CAD build for the part. Positions are in the model's coordinates, mm. A direction names the side the tool comes from. Give positions to 0.01 mm unless a question says otherwise; leave off trailing zeros. Loops run counter-clockwise (first coordinate to the right, second up) from the corner with the lowest first, then second, coordinate; pieces in that order, holes last. Notation, with made-up numbers: M 49.25,34 L 104.25,34 A22 ccw 104.25,52 Z; hole C 71.5,37 d2. An arc over 180 degrees is marked long. One line per question, with ' | ' between items.
```python
from build123d import *

# Parameters (mm, degrees)
F0_W      = 69.85
F0_H      = 76.2
F1_DEPTH  = 20.32
F2_R      = 5.08
F3_R      = 2.3749
F4_DEPTH  = 20.321
F5_R      = 10.0274789958
F6_DEPTH  = 8.128
F7_R      = 6.9469
F8_DEPTH  = 0.508
F10_DEPTH = 17.145
F11_R     = 10.9855
F12_DEPTH = 5.08
F11_R_2   = 5.08
F13_DEPTH = 6.35
F14_DEPTH = 6.35
F15_R     = 1.905
F16_DEPTH = 5.08
F18_R     = 1.927412261
F18_R_2   = 1.8880097215
F19_DEPTH = 3.048
F21_DEPTH = 76.2
F22_R     = 10.16
F23_DEPTH = 13.208
F25_DEPTH = 7.62
F27_DEPTH = 6.35


with BuildPart() as f1:
    # F0 (on Front) → F1 (new body)
    with BuildSketch(Plane.XZ):
        Rectangle(F0_W, F0_H)
    extrude(amount=F1_DEPTH)

    # F2
    f2_edges = [f1.edges().sort_by_distance(p)[0] for p in [
        (-34.925, -10.16, 38.1),
        (-34.925, -10.16, -38.1),
        (34.925, -10.16, -38.1),
        (34.925, -10.16, 38.1),
    ]]
    fillet(f2_edges, radius=F2_R)

    # F3 (on face) → F4 (cut, through all)
    with BuildSketch(Plane.XZ.offset(20.32)):
        with Locations((-29.845, 33.02)):
            Circle(F3_R)
        with Locations((29.845, 33.02)):
            Circle(F3_R)
        with Locations((-29.845, -33.02)):
            Circle(F3_R)
        with Locations((29.845, -33.02)):
            Circle(F3_R)
    extrude(amount=-F4_DEPTH, mode=Mode.SUBTRACT)

    # F5 (on face) → F6 (join)
    with BuildSketch(Plane.XZ.offset(20.32)):
        with Locations((0, 15.24)):
            Circle(F5_R)
    extrude(amount=F6_DEPTH)

    # F7 (on face) → F8 (cut)
    with BuildSketch(Plane.XZ.offset(28.448)):
        with Locations((0, 15.24)):
            Circle(F7_R)
    extrude(amount=-F8_DEPTH, mode=Mode.SUBTRACT)

    # F9 (on face) → F10 (join)
    with BuildSketch(Plane.XZ.offset(27.94)):
        with BuildLine():
            Line((2.3486417351, 18.4785), (-2.3486417351, 18.4785))
            ThreePointArc((-2.3486417351, 18.4785), (0, 11.2395), (2.3486417351, 18.4785))
        make_face()
    extrude(amount=F10_DEPTH)

    # F11 (on face) → F12 (join)
    with BuildSketch(Plane(origin=(0, 0, 0), x_dir=(-1, 0, 0), z_dir=(0, 1, 0))):
        with Locations((0, -22.86)):
            Circle(F11_R)
    extrude(amount=F12_DEPTH)

    # F11 (on face) → F13 (join)
    with BuildSketch(Plane(origin=(0, 0, 0), x_dir=(-1, 0, 0), z_dir=(0, 1, 0))):
        with Locations((26.035, -22.86)):
            Circle(F11_R_2)
    extrude(amount=F13_DEPTH)

    # F11 (on face) → F14 (join)
    with BuildSketch(Plane(origin=(0, 0, 0), x_dir=(-1, 0, 0), z_dir=(0, 1, 0))):
        with Locations((-26.035, -22.86)):
            Circle(F11_R_2)
    extrude(amount=F14_DEPTH)

    # F15 (on face) → F16 (cut)
    with BuildSketch(Plane(origin=(0, 5.08, 0), x_dir=(-1, 0, 0), z_dir=(0, 1, 0))):
        with Locations((0, -22.86)):
            Circle(F15_R)
    extrude(amount=-F16_DEPTH, mode=Mode.SUBTRACT)

    # F18 (on face) → F19 (join)
    with BuildSketch(Plane(origin=(0, 6.35, 0), x_dir=(-1, 0, 0), z_dir=(0, 1, 0))):
        with BuildLine():
            Line((-14.7449402664, -7.9254461452), (-28.5812491882, -19.9236759913))
            ThreePointArc((-28.5812491882, -19.9236759913), (-29.9214809801, -22.8854794861), (-28.5425313232, -25.8294562256))
            Line((-28.5425313232, -25.8294562256), (-14.7449402664, -37.4807112473))
            ThreePointArc((-14.7449402664, -37.4807112473), (0.0825790048, -43.6704553243), (14.9377645792, -37.5474069801))
            Line((14.9377645792, -37.5474069801), (28.3769337433, -25.961730155))
            ThreePointArc((28.3769337433, -25.961730155), (29.9185109104, -23.0140344812), (28.6152424237, -19.9535016519))
            Line((28.6152424237, -19.9535016519), (15.0339949064, -7.9553720766))
            ThreePointArc((15.0339949064, -7.9553720766), (0.1507626975, -1.7356597256), (-14.7449402664, -7.9254461452))
        make_face()
        with Locations((-26.035, -22.86)):
            Circle(F18_R, mode=Mode.SUBTRACT)
        with Locations((26.035, -22.86)):
            Circle(F18_R_2, mode=Mode.SUBTRACT)
    extrude(amount=F19_DEPTH)

    # F20 (on face) → F21 (join)
    with BuildSketch(Plane(origin=(0, 9.398, 0), x_dir=(-1, 0, 0), z_dir=(0, 1, 0))):
        with BuildLine():
            ThreePointArc((15.4071510025, -37.1427570095), (19.560406445, -30.5294042531), (21.0116482676, -22.8560827672))
            ThreePointArc((21.0116482676, -22.8560827672), (9.4227051618, -4.0757209402), (-12.5603957589, -6.0119199415))
            ThreePointArc((-12.5603957589, -6.0119199415), (-13.6858370585, -6.9308161687), (-14.7449402664, -7.9254461452))
            Line((-14.7449402664, -7.9254461452), (-15.0267070498, -8.16978173))
            ThreePointArc((-15.0267070498, -8.16978173), (-20.9946416555, -22.0108699669), (-16.15866039, -36.2869076608))
            Line((-16.15866039, -36.2869076608), (-14.7449402664, -37.4807112473))
            ThreePointArc((-14.7449402664, -37.4807112473), (0.0825790048, -43.6704553243), (14.9377645792, -37.5474069801))
            Line((14.9377645792, -37.5474069801), (15.4071510025, -37.1427570095))
        make_face()
    extrude(amount=F21_DEPTH)

    # F22 (on face) → F23 (join)
    with BuildSketch(Plane(origin=(0, 85.598, 0), x_dir=(-1, 0, 0), z_dir=(0, 1, 0))):
        with Locations((0.1296917782, -22.7030786963)):
            Circle(F22_R)
    extrude(amount=F23_DEPTH)

    # F24 (on face) → F25 (join)
    with BuildSketch(Plane(origin=(0, 85.598, 0), x_dir=(-1, 0, 0), z_dir=(0, 1, 0))):
        with BuildLine():
            Line((22.7089122915, -19.9516154365), (20.8099359068, -19.9516154365))
            ThreePointArc((20.8099359068, -19.9516154365), (21.0111071016, -22.7052806306), (20.8494821266, -25.4615497064))
            Line((20.8494821266, -25.4615497064), (22.7451570662, -25.4615497064))
            ThreePointArc((22.7451570662, -25.4615497064), (22.8934040546, -22.7054881808), (22.7089122915, -19.9516154365))
        make_face()
    extrude(amount=-F25_DEPTH)

    # F26 (on face) → F27 (join)
    with BuildSketch(Plane(origin=(0, 85.598, 0), x_dir=(-1, 0, 0), z_dir=(0, 1, 0))):
        with BuildLine():
            ThreePointArc((-20.8494821266, -25.4615497064), (-21.0115447656, -22.9220333613), (-20.8654271236, -20.3815497064))
            Line((-20.8654271236, -20.3815497064), (-22.4769224541, -20.3815497064))
            Line((-22.4769224541, -20.3815497064), (-22.4769224541, -25.4615497064))
            Line((-22.4769224541, -25.4615497064), (-20.8494821266, -25.4615497064))
        make_face()
    extrude(amount=-F27_DEPTH)


solid = f1.part
```
Item 1: 3-axis set-ups, long thin cutter, end or side, ignore diameter. For faces 4 (the flat face through (22.477, 82, -23)), 5 (the cylindrical face through (-22.894, 81.841, -22.744)), 6 (the flat face through (0, -10, -38.1)), 7 (the flat face through (-26, 6.35, -23)), 8 (the flat face through (0, -10, 38.1)): which of +Z, -Z, +X, -X, +Y, -Y reach the whole face in a straight line?
Conclusion:
face 4: +Z, -Z, +X, +Y | face 5: -X, +Y | face 6: -Z, +X, -X, -Y | face 7: +Y | face 8: +Z, +X, -X, +Y, -Y
Item 2: Saw through at C-C on z = 15.24. Give the cut face in (x, y) (1 decimal).
Conclusion:
outline: M -34.9,-20.3 L -10,-20.3 L -10,-28.4 L -6.9,-28.4 L -6.9,-27.9 L -4,-27.9 L -4,-45.1 L 4,-45.1 L 4,-27.9 L 6.9,-27.9 L 6.9,-28.4 L 10,-28.4 L 10,-20.3 L 34.9,-20.3 L 34.9,0 L -34.9,0 Z
Item 3: Saw through at D-D on y = 81.5. Give the cut face in (x, z).
Conclusion:
outline: M -22.75,-25.46 L -20.85,-25.46 A21.01 ccw -15.41,-37.14 L -14.94,-37.55 A20.97 ccw 14.74,-37.48 L 16.16,-36.29 A21.01 ccw 20.85,-25.46 L 22.48,-25.46 L 22.48,-20.38 L 20.87,-20.38 A21.01 ccw 15.03,-8.17 L 14.74,-7.93 A20.97 ccw 12.56,-6.01 A21.01 ccw -20.81,-19.95 L -22.71,-19.95 A22.89 ccw Z
Item 4: Saw through at A-A on x = 18.5. Give the cut face in (y, z).
Conclusion:
outline: M -20.32,-38.1 L 0,-38.1 L 0,38.1 L -20.32,38.1 Z; M 6.35,-34.31 L 9.4,-34.31 L 9.4,-32.82 L 85.6,-32.82 L 85.6,-12.89 L 9.4,-12.89 L 9.4,-11.18 L 6.35,-11.18 Z
Item 5: Drill centre lines: line 1 along X through (y, z) = (-12, 33) (3 decimals); line 2 along Y through (x, z) = (-9, -9.5); line 3 along Y through (x, z) = (-7, -18). Where is each one in solid material? Low to high. Write a range as [from, to].
Conclusion:
line 1: [-34.925, -32.22], [-27.47, 27.47], [32.22, 34.925] | line 2: [-20.32, 0], [6.35, 85.6] | line 3: [-20.32, 5.08], [6.35, 98.81]
Item 6: Saw through at B-B on y = 19. Give the cut face in (x, z), and give its area (3 significant figures).
Conclusion:
outline: M -15.41,-37.14 L -14.94,-37.55 A20.97 ccw 14.74,-37.48 L 16.16,-36.29 A21.01 ccw 15.03,-8.17 L 14.74,-7.93 A20.97 ccw 12.56,-6.01 A21.01 ccw Z | area: 1,380 mm²
Item 7: Mould opens along Y. For faces 1 (the cylindrical face through (33, -10, -37)), 2 (the flat face through (0, -20.32, 1)), 3 (the cylindrical face through (1.43, 2.504, -11.968)) say: pulls with the +Y half, pulls with the -Y half, needs draft (parallel to the pull), parting line crosses it, or undercut.
Conclusion:
face 1: needs draft | face 2: pulls with the -Y half | face 3: undercut
Item 8: Drop flat-ended pins along their axis: P1, Ø6, axis at x = -7.5, y = 58, coming from the -Z side; P2, Ø1.4, axis at x = 1, y = -34, coming from the +Z side; P3, Ø6, axis at x = 24, z = 11.5, coming from the -Y side. Give the stop position or say it passes through.
Conclusion:
P1: z = -43.21 | P2: z = 18.48 | P3: y = -20.32
